from build123d import *

# Parameters (mm, degrees)
EXTRUDE_1_DEPTH     = 4
SKETCH_12_R         = 4.75
SKETCH_12_R_2       = 10.958447214
CUT_EXTRUDE_1_DEPTH = 4
FILLET_1_R          = 10


with BuildPart() as part:
    # Sketch 1 → 凸台-拉伸1 (new body)
    with BuildSketch(Plane.XY):
        with BuildLine():
            ThreePointArc((-51.5, 0), (-53.628497347, 10.807120237), (-59.696059496, 20))
            ThreePointArc((-59.696059496, 20), (-108.5, 0), (-59.696059496, -20))
            ThreePointArc((-59.696059496, -20), (-53.628497347, -10.807120237), (-51.5, 0))
        make_face()
        with BuildLine():
            ThreePointArc((59.696059496, -20), (51.5, 0), (59.696059496, 20))
            Line((59.696059496, 20), (-59.696059496, 20))
            ThreePointArc((-59.696059496, 20), (-53.628497347, 10.807120237), (-51.5, 0))
            ThreePointArc((-51.5, 0), (-53.628497347, -10.807120237), (-59.696059496, -20))
            Line((-59.696059496, -20), (59.696059496, -20))
        make_face()
        with BuildLine():
            ThreePointArc((108.5, 0), (90.807120237, 26.371502653), (59.696059496, 20))
            ThreePointArc((59.696059496, 20), (51.5, 0), (59.696059496, -20))
            ThreePointArc((59.696059496, -20), (90.807120237, -26.371502653), (108.5, 0))
        make_face()
    extrude(amount=EXTRUDE_1_DEPTH)

    # 草图12 → 切除-拉伸1 (cut)
    with BuildSketch(Plane.XY.offset(4)):
        with Locations((-80, 0)):
            Circle(SKETCH_12_R)
        with Locations((80, 0)):
            Circle(SKETCH_12_R_2)
    extrude(amount=-CUT_EXTRUDE_1_DEPTH, mode=Mode.SUBTRACT)

    # 圆角1
    fillet_1_edges = [part.edges().sort_by_distance(p)[0] for p in [
        (-59.696059496, -20, 2),
        (59.696059496, -20, 2),
        (59.696059496, 20, 2),
        (-59.696059496, 20, 2),
    ]]
    fillet(fillet_1_edges, radius=FILLET_1_R)


solid = part.part
The model under review builds one solid part; all positions refer to its coordinate system, in mm. A direction names the side the tool comes from. Coordinates: 2 decimals unless noted, no trailing zeros. Loops run counter-clockwise (first coordinate to the right, second up) from the corner with the lowest first, then second, coordinate; pieces in that order, holes last. Notation, with made-up numbers: (81.25, -19) -> (112.25, -19) arc R13 ccw to (112.25, 6) -> close; hole circle Ø1 at (61, 86.5). An arc over 180 degrees is marked (long way). Use a Markdown table: item, result. Add a question column.
1. Add section A-A on x = -80. Write out the cut boundary in (y, z), plus the area to 3 significant figures.
2. Add section C-C on y = 8.5. Write out the cut boundary in (x, z), plus the area to 3 significant figures.
3. To check wall thickness, follow line 1 (Y direction, x = -80, z = 1.4); line 2 (Y direction, x = 80, z = 2.85); line 3 (X direction, y = 2.5, z = 2.9). State the ranges of each line that lie inside material, in increasing order.
4. Clearance check with flat-ended pins moving along their axes: pin 1 Ø2 at (x, z) = (-49, 2.5) entering from -Y; pin 2 Ø1.2 at (x, z) = (23, 2) entering from +Y. State where each tip first meets the part, or that it passes through.
5. Add section D-D on x = -19.5. Write out the cut boundary in (y, z).
6. Add section B-B on z = 2.3. Write out the cut boundary in (x, y), plus the area to 3 significant figures.
7. Machinability: for faces 4 (the face through (-2, 0, 0)), 5 (the face through (1, 20, 2)), 6 (the face through (-1, -20, 2)), which of the approach directions +Z, -Z, +X, -X, +Y, -Y give a long, thin tool a straight path to every point of the face, cutting with its end or side? Answer none if there is none.
8. Draft analysis for pull direction Y (two halves, no side actions). For faces 1 (the face through (-77.808, -4.214, 2.028)), 2 (the face through (-59.237, -20.584, 2.028)), 3 (the face through (-2, 0, 4)), state which applies: pulls with the +Y half, pulls with the -Y half, needs draft (parallel to the pull), parting line crosses it, or undercut.
Returned:
| question | item | result |
|---|---|---|
| 1 | outline | (-28.5, 0) -> (-4.75, 0) -> (-4.75, 4) -> (-28.5, 4) -> close; (4.75, 0) -> (28.5, 0) -> (28.5, 4) -> (4.75, 4) -> close |
| 1 | area | 190 mm² |
| 2 | outline | (-107.2, 0) -> (73.08, 0) -> (73.08, 4) -> (-107.2, 4) -> close; (86.92, 0) -> (107.2, 0) -> (107.2, 4) -> (86.92, 4) -> close |
| 2 | area | 802 mm² |
| 3 | line 1 | y = -28.5 to -4.75, 4.75 to 28.5 |
| 3 | line 2 | y = -28.5 to -10.96, 10.96 to 28.5 |
| 3 | line 3 | x = -108.39 to -84.04, -75.96 to 69.33, 90.67 to 108.39 |
| 4 | pin 1 | stops at y = -20 |
| 4 | pin 2 | stops at y = 20 |
| 5 | outline | (-20, 0) -> (20, 0) -> (20, 4) -> (-20, 4) -> close |
| 6 | outline | (-62.14, -22.21) arc R10 cw to (-55.87, -20) -> (55.87, -20) arc R10 cw to (62.14, -22.21) arc R28.5 ccw (long way) to (62.14, 22.21) arc R10 cw to (55.87, 20) -> (-55.87, 20) arc R10 cw to (-62.14, 22.21) arc R28.5 ccw (long way) to start; hole circle Ø9.5 at (-80, 0); hole circle Ø21.92 at (80, 0) |
| 6 | area | 8,990 mm² |
| 7 | face 4 | -Z, +X, -X, +Y, -Y |
| 7 | face 5 | +Z, -Z, +Y |
| 7 | face 6 | +Z, -Z, -Y |
| 8 | face 1 | undercut |
| 8 | face 2 | pulls with the -Y half |
| 8 | face 3 | needs draft |
